from build123d import *

# Parameters (mm, degrees)
SKETCH3_W           = 135
SKETCH3_H           = 118
BOSS_EXTRUDE1_DEPTH = 30
SKETCH4_W           = 131
SKETCH4_H           = 114
CUT_EXTRUDE1_DEPTH  = 28
SKETCH6_W           = 121
SKETCH6_H           = 70.2
SKETCH6_W_2         = 23
SKETCH6_H_2         = 11
SKETCH6_W_3         = 50
SKETCH6_H_3         = 30
BOSS_EXTRUDE2_DEPTH = 5
FILLET1_R           = 1
FILLET2_R           = 1
FILLET3_R           = 1
FILLET4_R           = 1


with BuildPart() as part:
    # Sketch3 → Boss-Extrude1 (new body)
    with BuildSketch(Plane(origin=(0, 0, 0), x_dir=(1, 0, 0), z_dir=(0, 1, 0))):
        Rectangle(SKETCH3_W, SKETCH3_H)
    extrude(amount=BOSS_EXTRUDE1_DEPTH)

    # Sketch4 → Cut-Extrude1 (cut)
    with BuildSketch(Plane(origin=(0, 30, 0), x_dir=(1, 0, 0), z_dir=(0, 1, 0))):
        Rectangle(SKETCH4_W, SKETCH4_H)
    extrude(amount=-CUT_EXTRUDE1_DEPTH, mode=Mode.SUBTRACT)

    # Sketch6 → Boss-Extrude2 (add)
    with BuildSketch(Plane(origin=(0, 2, 0), x_dir=(1, 0, 0), z_dir=(0, 1, 0))):
        with Locations((-0.543145458, 17.603777785)):
            Rectangle(SKETCH6_W, SKETCH6_H)
        with Locations((-37.163103621, -38.689582539)):
            Rectangle(SKETCH6_W_2, SKETCH6_H_2)
        with Locations((15.455951062, -38.689582539)):
            Rectangle(SKETCH6_W_3, SKETCH6_H_3)
    extrude(amount=BOSS_EXTRUDE2_DEPTH)

    # Fillet1
    fillet1_edges = [part.edges().sort_by_distance(p)[0] for p in [
        (-67.5, 15, 59),
    ]]
    fillet(fillet1_edges, radius=FILLET1_R)

    # Fillet2
    fillet2_edges = [part.edges().sort_by_distance(p)[0] for p in [
        (67.5, 15, 59),
    ]]
    fillet(fillet2_edges, radius=FILLET2_R)

    # Fillet3
    fillet3_edges = [part.edges().sort_by_distance(p)[0] for p in [
        (67.5, 15, -59),
    ]]
    fillet(fillet3_edges, radius=FILLET3_R)

    # Fillet4
    fillet4_edges = [part.edges().sort_by_distance(p)[0] for p in [
        (-67.5, 15, -59),
    ]]
    fillet(fillet4_edges, radius=FILLET4_R)


solid = part.part
Work out the finished part from the listing and answer in its coordinate system (mm). A direction names the side the tool comes from. Round coordinates to 2 decimals unless told otherwise and drop trailing zeros. Order: outer loops, then holes, each group sorted by start corner. A loop starts at its lowest first (then second) coordinate and runs counter-clockwise, first axis right, second up. Notation, with made-up numbers: M -23,70 L 14,70 A18 ccw 14,103 Z; hole C -19,62.25 d4. An arc over 180 degrees is marked long. One line per item, written item: value.
Q1. Find section C-C on x = -16.5. Write down the section's boundary in (y, z).
Derived:
outline: M 0,-59 L 30,-59 L 30,-57 L 2,-57 L 2,-52.7 L 7,-52.7 L 7,17.5 L 2,17.5 L 2,57 L 30,57 L 30,59 L 0,59 Z
Q2. For faces 1 (the face through (-67.5, 15, 1)), 2 (the face through (59.957, 4, -17)), determine the directions among +Z, -Z, +X, -X, +Y, -Y from which every point of the face is accessible in a straight line to the end or side of a thin tool.
Derived:
face 1: +Z, -Z, -X, +Y, -Y
face 2: +Y
Q3. Determine the mould class of faces 3 (the face through (-1, 0, -1)), 4 (the face through (-1, 15, -59)), 5 (the face through (-25.663, 4, 39)) for opening direction Z: released by +Z, released by -Z, zero draft, split by the parting line, or undercut.
Derived:
face 3: zero draft
face 4: released by -Z
face 5: undercut
Q4. Straight lines are drawn through the part: line 1 (X direction, y = 6.5, z = 2); line 2 (Z direction, x = 11, y = 3.25); line 3 (Z direction, x = 21, y = 8.25). For each, find the intervals that lie inside material, in ascending order.
Derived:
line 1: -67.5 to -65.5, -61.04 to 59.96, 65.5 to 67.5
line 2: -59 to -57, -52.7 to 17.5, 23.69 to 53.69, 57 to 59
line 3: -59 to -57, 57 to 59
Q5. A flat-ended cylindrical pin translates along its axis: pin 1 (3.5 mm diameter, centred on x = -38, z = 36.5, fed in from +Y). Find the tip coordinate at first contact, or state that the pin passes through.
Derived:
pin 1: y = 7
Q6. Find section D-D on z = -20. Write down the section's boundary in (x, y), then the cut area to 3 significant figures.
Derived:
outline: M -67.5,0 L 67.5,0 L 67.5,30 L 65.5,30 L 65.5,2 L 59.96,2 L 59.96,7 L -61.04,7 L -61.04,2 L -65.5,2 L -65.5,30 L -67.5,30 Z
area: 987 mm²
Q7. Find section A-A on y = 28. Write down the section's boundary in (x, z).
Derived:
outline: M -67.5,-58 A1 ccw -66.5,-59 L 66.5,-59 A1 ccw 67.5,-58 L 67.5,58 A1 ccw 66.5,59 L -66.5,59 A1 ccw -67.5,58 Z; hole M -65.5,-57 L 65.5,-57 L 65.5,57 L -65.5,57 Z
Q8. Find section B-B on z = 38. Write down the section's boundary in (x, y), then the cut area to 3 significant figures.
Derived:
outline: M -67.5,0 L 67.5,0 L 67.5,30 L 65.5,30 L 65.5,2 L 40.46,2 L 40.46,7 L -9.54,7 L -9.54,2 L -25.66,2 L -25.66,7 L -48.66,7 L -48.66,2 L -65.5,2 L -65.5,30 L -67.5,30 Z
area: 747 mm²
